```python
from build123d import *

# Parameters (mm, degrees)
CUT_EXTRUDE_1_REACH      = 76.218
SKETCH_5_R               = 1.75
PATTERN_CIRCULAR_2_COUNT = 12
SKETCH_9_R               = 22.5
SKETCH_9_R_2             = 10
EXTRUDE_1_DEPTH          = 5.5
PATTERN_CIRCULAR_4_COUNT = 3
SKETCH_12_R              = 14
SKETCH_12_R_2            = 12.5
CUT_EXTRUDE_4_DEPTH      = 0.5
CUT_EXTRUDE_START        = -0.5
SKETCH_14_R              = 14
SKETCH_14_R_2            = 12.5
CUT_EXTRUDE_5_DEPTH      = 0.5
PATTERN_CIRCULAR_5_COUNT = 4
PATTERN_CIRCULAR_5_ANGLE = 54
PATTERN_CIRCULAR_6_COUNT = 4
PATTERN_CIRCULAR_7_COUNT = 4


with BuildPart() as part:
    # Sketch 1 → Revolve 1 (revolve)
    with BuildSketch(Plane.XY, mode=Mode.PRIVATE) as revolve_1_sk:
        Polygon((0, 9.5), (0, 12.5), (12, 12.5), (12, 42), (22, 42), (22, 40), (35, 40), (35, 32), (39.5, 29.401923789), (39.5, 32), (48, 32), (48, 22.5), (56.5, 22.5), (56.5, 9.5), align=None)
    revolve(revolve_1_sk.sketch.rotate(Axis((-65.200779727, 0, 0), (1, 0, 0)), 90), axis=Axis((-65.200779727, 0, 0), (1, 0, 0)))

    # Sketch 5 → Cut-Extrude 1 (cut, up to next)
    with BuildSketch(Plane.ZY.offset(-12), mode=Mode.PRIVATE) as cut_extrude_1_sk1:
        with Locations((0, 37)):
            Circle(SKETCH_5_R)
    cut_extrude_1_tool1 = extrude(cut_extrude_1_sk1.sketch, amount=-CUT_EXTRUDE_1_REACH, mode=Mode.PRIVATE) & part.part
    cut_extrude_1 = cut_extrude_1_tool1.solids().sort_by_distance((12, 37, 0))[0]
    add(cut_extrude_1, mode=Mode.SUBTRACT)

    # Pattern Circular 2: Cut-Extrude 1 ×12 about axis
    pattern_circular_2_axis = Axis((0, 0, 0), (1, 0, 0))
    for i in range(1, PATTERN_CIRCULAR_2_COUNT):
        add(cut_extrude_1.rotate(pattern_circular_2_axis, i * 360 / PATTERN_CIRCULAR_2_COUNT), mode=Mode.SUBTRACT)

    # Sketch 9 → Extrude 1 (add)
    with BuildSketch(Plane.ZY.offset(-12)):
        Circle(SKETCH_9_R)
        Circle(SKETCH_9_R_2, mode=Mode.SUBTRACT)
    extrude(amount=EXTRUDE_1_DEPTH)

    # Sketch 10 → Hole Wizard M3 _3 (revolve, cut)
    with BuildSketch(Plane(origin=(2.5, 12.5, 0), x_dir=(0, 0, 1), z_dir=(1, 0, 0))):
        Polygon((0, 0), (0, 7.251075774), (1.25, 6.5), (1.25, 0), align=None)
    hole_wizard_m3_3 = revolve(axis=Axis((2.5, 18.85, 0), (0, -1, 0)), mode=Mode.SUBTRACT)

    # Pattern Circular 4: Hole Wizard M3 _3 ×3 about axis
    pattern_circular_4_axis = Axis((56.5, 0, 0), (-1, 0, 0))
    for i in range(1, PATTERN_CIRCULAR_4_COUNT):
        add(hole_wizard_m3_3.rotate(pattern_circular_4_axis, i * 360 / PATTERN_CIRCULAR_4_COUNT), mode=Mode.SUBTRACT)

    # Sketch 12 → Cut-Extrude 4 (cut)
    with BuildSketch(Plane(origin=(56.5, 0, 0), x_dir=(0, 0, -1), z_dir=(1, 0, 0))):
        Circle(SKETCH_12_R)
        with Locations(Location((0, 0, 0), (0, 0, 180))):
            Circle(SKETCH_12_R_2, mode=Mode.SUBTRACT)
    extrude(amount=-CUT_EXTRUDE_4_DEPTH, mode=Mode.SUBTRACT)

    # Sketch 14 → Cut-Extrude 5 (cut)
    with BuildSketch(Plane.ZY.offset(-6.5).offset(CUT_EXTRUDE_START)):
        with Locations(Location((0, 0, 0), (0, 0, 180))):
            Circle(SKETCH_14_R)
        Circle(SKETCH_14_R_2, mode=Mode.SUBTRACT)
    extrude(amount=CUT_EXTRUDE_5_DEPTH, mode=Mode.SUBTRACT)

    # Sketch 15 → Hole Wizard M3 _4 (revolve, cut)
    with BuildSketch(Plane(origin=(48, 27, 0), x_dir=(0, 0, -1), z_dir=(0, 1, 0))):
        Polygon((0, 0), (0, 12.751075774), (1.25, 12), (1.25, 0), align=None)
    hole_wizard_m3_4 = revolve(axis=Axis((54.35, 27, 0), (-1, 0, 0)), mode=Mode.SUBTRACT)

    # Pattern Circular 5: Hole Wizard M3 _4 ×4 about axis
    pattern_circular_5_axis = Axis((0, 0, 0), (-1, 0, 0))
    for i in range(1, PATTERN_CIRCULAR_5_COUNT):
        add(hole_wizard_m3_4.rotate(pattern_circular_5_axis, i * PATTERN_CIRCULAR_5_ANGLE / (PATTERN_CIRCULAR_5_COUNT - 1)), mode=Mode.SUBTRACT)

    # Pattern Circular 6: Hole Wizard M3 _4 ×4 about axis
    pattern_circular_6_axis = Axis((0, 0, 0), (1, 0, 0))
    for i in range(1, PATTERN_CIRCULAR_6_COUNT):
        add(hole_wizard_m3_4.rotate(pattern_circular_6_axis, i * 360 / PATTERN_CIRCULAR_6_COUNT), mode=Mode.SUBTRACT)

    # Pattern Circular 6 copy 1 sketch → Pattern Circular 6 copy 1 (revolve, cut)
    with BuildSketch(Plane(origin=(48, 8.343458848, 25.67852594), x_dir=(0, 0.9510565162951534, -0.3090169943749481), z_dir=(0, 0.3090169943749481, 0.9510565162951534))):
        Polygon((0, 0), (0, 12.751075774), (1.25, 12), (1.25, 0), align=None)
    revolve(axis=Axis((54.35, 8.343458848, 25.67852594), (-1, 0, 0)), mode=Mode.SUBTRACT)

    # Pattern Circular 6 copy 2 sketch → Pattern Circular 6 copy 2 (revolve, cut)
    with BuildSketch(Plane(origin=(48, -25.67852594, 8.343458848), x_dir=(0, 0.3090169943749482, 0.9510565162951534), z_dir=(0, -0.9510565162951534, 0.3090169943749482))):
        Polygon((0, 0), (0, 12.751075774), (1.25, 12), (1.25, 0), align=None)
    revolve(axis=Axis((54.35, -25.67852594, 8.343458848), (-1, 0, 0)), mode=Mode.SUBTRACT)

    # Pattern Circular 6 copy 3 sketch → Pattern Circular 6 copy 3 (revolve, cut)
    with BuildSketch(Plane(origin=(48, -8.343458848, -25.67852594), x_dir=(0, -0.9510565162951533, 0.30901699437494823), z_dir=(0, -0.30901699437494823, -0.9510565162951533))):
        Polygon((0, 0), (0, 12.751075774), (1.25, 12), (1.25, 0), align=None)
    revolve(axis=Axis((54.35, -8.343458848, -25.67852594), (-1, 0, 0)), mode=Mode.SUBTRACT)

    # Pattern Circular 6 copy 4 sketch → Pattern Circular 6 copy 4 (revolve, cut)
    with BuildSketch(Plane(origin=(48, 15.870201812, 21.843458848), x_dir=(0, 0.8090169943749467, -0.5877852522924741), z_dir=(0, 0.5877852522924741, 0.8090169943749467))):
        Polygon((0, 0), (0, 12.751075774), (1.25, 12), (1.25, 0), align=None)
    revolve(axis=Axis((54.35, 15.870201812, 21.843458848), (-1, 0, 0)), mode=Mode.SUBTRACT)

    # Pattern Circular 6 copy 5 sketch → Pattern Circular 6 copy 5 (revolve, cut)
    with BuildSketch(Plane(origin=(48, -21.843458848, 15.870201812), x_dir=(0, 0.5877852522924742, 0.8090169943749466), z_dir=(0, -0.8090169943749466, 0.5877852522924742))):
        Polygon((0, 0), (0, 12.751075774), (1.25, 12), (1.25, 0), align=None)
    revolve(axis=Axis((54.35, -21.843458848, 15.870201812), (-1, 0, 0)), mode=Mode.SUBTRACT)

    # Pattern Circular 6 copy 6 sketch → Pattern Circular 6 copy 6 (revolve, cut)
    with BuildSketch(Plane(origin=(48, -15.870201812, -21.843458848), x_dir=(0, -0.8090169943749466, 0.5877852522924742), z_dir=(0, -0.5877852522924742, -0.8090169943749466))):
        Polygon((0, 0), (0, 12.751075774), (1.25, 12), (1.25, 0), align=None)
    revolve(axis=Axis((54.35, -15.870201812, -21.843458848), (-1, 0, 0)), mode=Mode.SUBTRACT)

    # Pattern Circular 6 copy 7 sketch → Pattern Circular 6 copy 7 (revolve, cut)
    with BuildSketch(Plane(origin=(48, 21.843458848, 15.870201812), x_dir=(0, 0.5877852522924716, -0.8090169943749486), z_dir=(0, 0.8090169943749486, 0.5877852522924716))):
        Polygon((0, 0), (0, 12.751075774), (1.25, 12), (1.25, 0), align=None)
    revolve(axis=Axis((54.35, 21.843458848, 15.870201812), (-1, 0, 0)), mode=Mode.SUBTRACT)

    # Pattern Circular 6 copy 8 sketch → Pattern Circular 6 copy 8 (revolve, cut)
    with BuildSketch(Plane(origin=(48, -15.870201812, 21.843458848), x_dir=(0, 0.8090169943749487, 0.5877852522924715), z_dir=(0, -0.5877852522924715, 0.8090169943749487))):
        Polygon((0, 0), (0, 12.751075774), (1.25, 12), (1.25, 0), align=None)
    revolve(axis=Axis((54.35, -15.870201812, 21.843458848), (-1, 0, 0)), mode=Mode.SUBTRACT)

    # Pattern Circular 6 copy 9 sketch → Pattern Circular 6 copy 9 (revolve, cut)
    with BuildSketch(Plane(origin=(48, -21.843458848, -15.870201812), x_dir=(0, -0.5877852522924715, 0.8090169943749487), z_dir=(0, -0.8090169943749487, -0.5877852522924715))):
        Polygon((0, 0), (0, 12.751075774), (1.25, 12), (1.25, 0), align=None)
    revolve(axis=Axis((54.35, -21.843458848, -15.870201812), (-1, 0, 0)), mode=Mode.SUBTRACT)

    # Sketch 17 → Hole Wizard 1 (revolve, cut)
    with BuildSketch(Plane(origin=(48, 25.67852594, 8.343458848), x_dir=(0, 0, -1), z_dir=(0, 1, 0))):
        Polygon((0, 0), (0, 16.521463052), (1.7, 15.5), (1.7, 3.4), (3, 3.4), (3, 0), align=None)
    hole_wizard_1 = revolve(axis=Axis((54.35, 25.67852594, 8.343458848), (-1, 0, 0)), mode=Mode.SUBTRACT)

    # Pattern Circular 7: Hole Wizard 1 ×4 about axis
    pattern_circular_7_axis = Axis((0, 0, 0), (1, 0, 0))
    for i in range(1, PATTERN_CIRCULAR_7_COUNT):
        add(hole_wizard_1.rotate(pattern_circular_7_axis, i * 360 / PATTERN_CIRCULAR_7_COUNT), mode=Mode.SUBTRACT)


solid = part.part
```
Could you check a few things on this model? Use its own coordinates, in mm. A direction names the side the tool comes from. Round coordinates to 2 decimals unless told otherwise and drop trailing zeros. Write each loop counter-clockwise with the first axis right and the second up, starting at its lowest first coordinate (ties: lowest second). Pieces come first, ordered by that corner, then holes. Notation, with made-up numbers: M -39.75,9 L -25.75,9 A23 ccw -25.75,20 Z; hole C -6.5,80.25 d1. An arc over 180 degrees is marked long. Write each question's results on one line, items separated by ' | '. Start each with the question number.
1. I'm going to push flat-ended pins straight in: pin 1 Ø2 at (y, z) = (0, 27) entering from +X; pin 2 Ø3 at (x, z) = (25, -6.5) entering from -Y; pin 3 Ø4.5 at (y, z) = (-8.34, 25.68) entering from -X; pin 4 Ø3 at (y, z) = (37, 0) entering from -X. Where does each tip first touch, or does it pass through?
2. On a 3-axis mill with a long thin cutter (end or side, diameter ignored), from which of +Z, -Z, +X, -X, +Y, -Y can I reach the whole of each face in a straight line? I mean faces 4 (the face through (46.32, -8.99, 28.61)), 5 (the face through (12, 18, -18)), 6 (the face through (39.282, 28.826, -6.401)). Say none if no direction works.
3. Thinking about a two-plate mould opening in Z: for faces 1 (the face through (48, -7.3, -21.5)), 2 (the face through (44.6, 27, 10)), 3 (the face through (23.34, -17.32, 30.75)), which applies, +Z half, -Z half, draft (parallel to the pull), parting line (faces both ways), or undercut?
4. I need wall thicknesses on L1, parallel to Y at x = 25, z = 0; L2, parallel to Y at x = 54, z = 0; L3, parallel to Y at x = 25, z = 32. Which ranges of each line are inside material? Lowest first, please. Write a range as from..to.
5. Imagine slicing it at B-B on x = 2.5. List the corners of the cut face in (y, z) for me, and give its area (3 significant figures).
6. Imagine slicing it at A-A on y = -37. List the corners of the cut face in (x, z) for me, and give its area (3 significant figures).
7. Imagine slicing it at D-D on x = 28.5. Count the separate pieces of the cut face and the enclosed holes in it, and give its area (3 significant figures).
Result sheet:
1) pin 1: stops at x = 35.85 | pin 2: stops at y = -39.69 | pin 3: stops at x = 12 | pin 4: passes through
2) face 4: +X | face 5: -X | face 6: none
3) face 1: draft | face 2: undercut | face 3: undercut
4) L1: y = -40..-38.75, -35.25..-9.5, 9.5..35.25, 38.75..40 | L2: y = -22.5..-9.5, 9.5..22.5 | L3: y = -24..-20.25, -16.75..16.75, 20.25..24
5) outline: M -7.3,-10.15 L -5.79,-7.53 A9.5 cw -5.79,7.53 L -7.3,10.15 A12.5 ccw Z; M -5.14,-11.4 A12.5 ccw 12.44,-1.25 L 9.42,-1.25 A9.5 cw -3.63,-8.78 Z; M -5.14,11.4 L -3.63,8.78 A9.5 cw 9.42,1.25 L 12.44,1.25 A12.5 ccw Z | area: 185 mm^2
6) outline: M 12,-19.87 L 22,-19.87 L 22,-15.2 L 35,-15.2 L 35,-1.75 L 12,-1.75 Z; M 12,1.75 L 35,1.75 L 35,15.2 L 22,15.2 L 22,19.87 L 12,19.87 Z | area: 712 mm^2
7) separate pieces: 1 | enclosed holes: 13 | area: 4,630 mm^2
